Check sheet for the modelled part. Datum: model origin and axes. Units: mm. A direction names the side the tool comes from. Coordinates: 2 decimals unless noted, no trailing zeros. Loops run counter-clockwise (first coordinate to the right, second up) from the corner with the lowest first, then second, coordinate; pieces in that order, holes last.
```python
from build123d import *

# Parameters (mm, degrees)
SKETCH006_R     = 2.75
PAD003_DEPTH    = 3
SKETCH007_R     = 1.5
PAD004_DEPTH    = 20
POCKET002_DEPTH = 4
CHAMFER004_SIZE = 0.2


with BuildPart() as part:
    # Sketch006 → Pad003 (new body)
    with BuildSketch(Plane.XY):
        Circle(SKETCH006_R)
    extrude(amount=PAD003_DEPTH)

    # Sketch007 (on Face2 of Pad003) → Pad004 (join)
    with BuildSketch(Plane(origin=(0, 0, 0), x_dir=(1, 0, 0), z_dir=(0, 0, -1))):
        Circle(SKETCH007_R)
    extrude(amount=PAD004_DEPTH)

    # Sketch008 (on DatumPlane) → Pocket002 (cut)
    with BuildSketch(Plane.XY.offset(3)):
        Polygon((0.721688, -1.25), (1.443376, 0), (0.721688, 1.25), (-0.721688, 1.25), (-1.443376, 0), (-0.721688, -1.25), align=None)
    extrude(amount=-POCKET002_DEPTH, mode=Mode.SUBTRACT)

    # Chamfer004
    chamfer004_edges = [part.edges().sort_by_distance(p)[0] for p in [
        (-1.5, 0, -20),
        (-2.75, 0, 0),
        (-2.75, 0, 3),
    ]]
    chamfer(chamfer004_edges, length=CHAMFER004_SIZE)


solid = part.part
```
1) Section check A-A on z = 1.75. Enter the section's corners in (x, y), plus the area to 3 significant figures.
Answer sheet:
outline: circle Ø5.5 at (0, 0); hole (-1.44, 0) - (-0.72, -1.25) - (0.72, -1.25) - (1.44, 0) - (0.72, 1.25) - (-0.72, 1.25) - close
area: 18.3 mm2
2) Section check B-B on x = 0. Enter the section's corners in (y, z), plus the area to 3 significant figures.
Answer sheet:
outline: (-2.75, 0.2) - (-2.55, 0) - (-1.5, 0) - (-1.5, -19.8) - (-1.3, -20) - (1.3, -20) - (1.5, -19.8) - (1.5, 0) - (2.55, 0) - (2.75, 0.2) - (2.75, 2.8) - (2.55, 3) - (1.25, 3) - (1.25, -1) - (-1.25, -1) - (-1.25, 3) - (-2.55, 3) - (-2.75, 2.8) - close
area: 66.4 mm2
3) Depth check by flat-ended pin: pin 1 (1.5 mm diameter, centred on y = 0.5, z = -1.5, fed in from -X). Enter the tip coordinate at first touch or a pass-through.
Answer sheet:
pin 1: stops at x = -1.5
4) Set-up check for faces 1 (the flat face through (0, -2, 0)), 2 (the flat face through (1.08, -0.63, 1.03)), 3 (the cylindrical face through (-0.596, -2.685, 1.482)): record each of +Z, -Z, +X, -X, +Y, -Y from which the full face is reachable in a straight line by a thin tool's end or side.
Answer sheet:
face 1: -Z
face 2: +Z
face 3: +Z, -Z
5) Mould release check, pull along X, two halves, no side actions. Record for faces 4 (the flat face through (1.088, 0.616, 1.028)), 5 (the flat face through (0, 0, -20)), 6 (the cylindrical face through (-1.5, -0.07, -9.76)): +X half, -X half, draft (parallel to the pull), parting line (faces both ways), or undercut.
Answer sheet:
face 4: undercut
face 5: draft
face 6: parting line
6) Section check C-C on z = -11.5. Enter the section's corners in (x, y).
Answer sheet:
outline: circle Ø3 at (0, 0)
7) Scan lines: line 1 (Z direction, x = -0.9, y = 0); line 2 (Y direction, x = 0.05, z = -4); line 3 (Z direction, x = 0.65, y = 1.95). Record each from-to range of solid material in increasing order.
Answer sheet:
line 1: z = -20 to -1
line 2: y = -1.5 to 1.5
line 3: z = 0 to 3
